Geometry check sheet. Reference: the model listing, model coordinates, mm. Face numbers are marked on the shaded views. Round coordinates to 2 decimals unless told otherwise and drop trailing zeros. Loops run counter-clockwise (first coordinate to the right, second up) from the corner with the lowest first, then second, coordinate; pieces in that order, holes last. Notation, with made-up numbers: (15, 62.5) - (30, 62.5) arc R10 ccw to (30, 75.5) - close; hole circle Ø1 at (88, 1.5). An arc over 180 degrees is marked (long way). Answer in a Markdown table with one row per item. Add a question column.
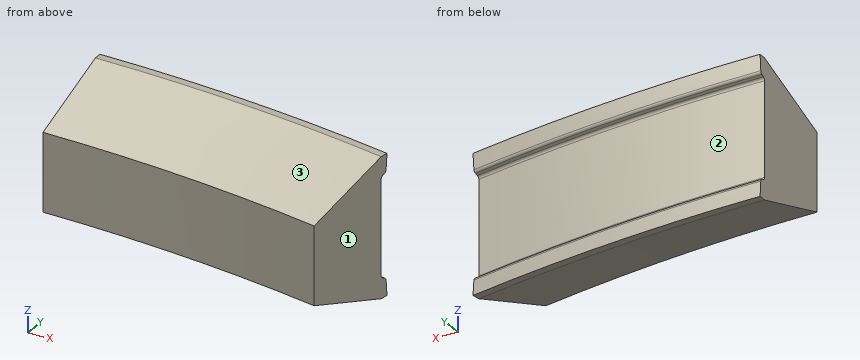
```python
from build123d import *

# Parameters (mm, degrees)
CROQUIS2_R                        = 2.1
CORTAR_EXTRUIR1_DEPTH             = 406.488213274
MATRIZC1_COUNT                    = 36
CORTAR_EXTRUIR5_REACH             = 679.172
CROQUIS4_R                        = 4.2
CORTAR_EXTRUIR5_DIRECTION_2_REACH = 679.172
REVOLUCI_N3_ANGLE                 = 10


with BuildPart() as part:
    # Croquis1 → Revolución2 (revolve)
    with BuildSketch(Plane(origin=(0, 0, 0), x_dir=(0, 0, -1), z_dir=(1, 0, 0)), mode=Mode.PRIVATE) as revoluci_n2_sk:
        with BuildLine():
            Line((-7.932667948, 272.794817661), (-8.128235692, 273.229412649))
            ThreePointArc((-8.128235692, 273.229412649), (-8.296797496, 273.433378016), (-8.545848195, 273.522757553))
            Line((-8.545848195, 273.522757553), (-12.682817286, 273.840985945))
            ThreePointArc((-12.682817286, 273.840985945), (-14.22986011, 274.537339899), (-14.976158002, 276.060917854))
            Line((-14.976158002, 276.060917854), (-16, 285.390918278))
            ThreePointArc((-16, 285.390918278), (-14.380212317, 286.280019748), (-14.896885493, 284.505967215))
            Line((-14.896885493, 284.505967215), (-14.369495262, 279.7))
            ThreePointArc((-14.369495262, 279.7), (-11.00403892, 278.246015718), (-9.3, 275))
            ThreePointArc((-9.3, 275), (-4.661345964, 274.499260763), (0, 274.3))
            ThreePointArc((0, 274.3), (4.661345964, 274.499260763), (9.3, 275))
            ThreePointArc((9.3, 275), (11.00403892, 278.246015718), (14.369495262, 279.7))
            Line((14.369495262, 279.7), (14.896885493, 284.505967215))
            ThreePointArc((14.896885493, 284.505967215), (14.380212317, 286.280019748), (16, 285.390918278))
            Line((16, 285.390918278), (14.976158002, 276.060917854))
            ThreePointArc((14.976158002, 276.060917854), (14.22986011, 274.537339899), (12.682817286, 273.840985945))
            Line((12.682817286, 273.840985945), (8.545848195, 273.522757553))
            ThreePointArc((8.545848195, 273.522757553), (8.296797496, 273.433378016), (8.128235692, 273.229412649))
            Line((8.128235692, 273.229412649), (7.932667948, 272.794817661))
            ThreePointArc((7.932667948, 272.794817661), (7.748192766, 272.580124322), (7.476707195, 272.5))
            Line((7.476707195, 272.5), (-7.476707195, 272.5))
            ThreePointArc((-7.476707195, 272.5), (-7.748192766, 272.580124322), (-7.932667948, 272.794817661))
        make_face()
    revolve(revoluci_n2_sk.sketch.rotate(Axis((0, 0, 417.631684514), (0, 0, -1)), 180), axis=Axis((0, 0, 417.631684514), (0, 0, -1)))

    # Croquis2 → Cortar-Extruir1 (cut, through all)
    with BuildSketch(Plane(origin=(0, 0, 0), x_dir=(1, 0, 0), z_dir=(0, 1, 0))):
        with Locations(Location((0, 0, 0), (0, 0, 270))):
            Circle(CROQUIS2_R)
    cortar_extruir1 = extrude(amount=-CORTAR_EXTRUIR1_DEPTH, mode=Mode.SUBTRACT)

    # MatrizC1: Cortar-Extruir1 ×36 about axis
    matrizc1_axis = Axis((0, 0, 0), (0, 0, 1))
    for i in range(1, MATRIZC1_COUNT):
        add(cortar_extruir1.rotate(matrizc1_axis, i * 360 / MATRIZC1_COUNT), mode=Mode.SUBTRACT)

    # Croquis4 → Cortar-Extruir5 (cut, up to next)
    with BuildSketch(Plane(origin=(-224.693405748, 157.332016491, 0), x_dir=(0, 0, -1), z_dir=(-0.8191520442889971, 0.5735764363510386, 0)), mode=Mode.PRIVATE) as cortar_extruir5_sk1:
        Circle(CROQUIS4_R)
    cortar_extruir5_tool1 = extrude(cortar_extruir5_sk1.sketch, amount=-CORTAR_EXTRUIR5_REACH, mode=Mode.PRIVATE) & part.part
    add(cortar_extruir5_tool1.solids().sort_by_distance((-224.693406, 157.332016, 0))[0], mode=Mode.SUBTRACT)

    # Croquis4 → Cortar-Extruir5 direction 2 (cut, up to next)
    with BuildSketch(Plane(origin=(-224.693405748, 157.332016491, 0), x_dir=(0, 0, -1), z_dir=(-0.8191520442889971, 0.5735764363510386, 0)), mode=Mode.PRIVATE) as cortar_extruir5_direction_2_sk1:
        Circle(CROQUIS4_R)
    cortar_extruir5_direction_2_tool1 = extrude(cortar_extruir5_direction_2_sk1.sketch, amount=CORTAR_EXTRUIR5_DIRECTION_2_REACH, mode=Mode.PRIVATE) & part.part
    add(cortar_extruir5_direction_2_tool1.solids().sort_by_distance((-224.693406, 157.332016, 0))[0], mode=Mode.SUBTRACT)


with BuildPart() as body_2:
    # Croquis5 → Revolución3 (revolve)
    with BuildSketch(Plane(origin=(0, 0, 0), x_dir=(0, 0, -1), z_dir=(1, 0, 0))):
        with BuildLine():
            Line((-11, 273.711538462), (-11, 272.5))
            Line((-11, 272.5), (-7.476707195, 272.5))
            ThreePointArc((-7.476707195, 272.5), (-7.748192766, 272.580124322), (-7.932667948, 272.794817661))
            Line((-7.932667948, 272.794817661), (-8.128235692, 273.229412649))
            ThreePointArc((-8.128235692, 273.229412649), (-8.296797496, 273.433378016), (-8.545848195, 273.522757553))
            Line((-8.545848195, 273.522757553), (-11, 273.711538462))
        make_face()
        Polygon((-7.476707195, 272.5), (-11, 272.5), (-6.179413414, 258.5), (0, 258.5), (0, 272.5), align=None)
        Polygon((7.476707195, 272.5), (0, 272.5), (0, 258.5), (6.179413414, 258.5), (11, 272.5), align=None)
        with BuildLine():
            ThreePointArc((7.932667948, 272.794817661), (7.748192766, 272.580124322), (7.476707195, 272.5))
            Line((7.476707195, 272.5), (11, 272.5))
            Line((11, 272.5), (11, 273.711538462))
            Line((11, 273.711538462), (8.545848195, 273.522757553))
            ThreePointArc((8.545848195, 273.522757553), (8.296797496, 273.433378016), (8.128235692, 273.229412649))
            Line((8.128235692, 273.229412649), (7.932667948, 272.794817661))
        make_face()
    revolve(axis=Axis((0, 0, 417.631684514), (0, 0, -1)), revolution_arc=REVOLUCI_N3_ANGLE)


solid = body_2.part
```
Q1. Scan lines: line 1 (Z direction, x = 21, y = 271.75); line 2 (Z direction, x = 13, y = 266.5); line 3 (Z direction, x = 2, y = 265.75). Record each from-to range of solid material in increasing order. Write a range as from..to.
Q2. Depth check by flat-ended pin: P1, Ø2, axis at x = 37.5, y = 268.5, coming from the -Z side; P2, Ø4, axis at y = 261.5, z = 6.5, coming from the +X side; P3, Ø4, axis at y = 259.5, z = -0.5, coming from the +X side. Enter the tip coordinate at first touch or a pass-through.
Q3. Release check for a two-part mould opening along Z. For the marked faces 1, 2 and 3 record: +Z half, -Z half, draft (parallel to the pull), parting line (faces both ways), or undercut.
Q4. Cross-section at A-A, the plane z = -0.5. Enter the section's corners in (x, y), plus the area to 3 significant figures.
Check sheet entries:
| question | item | result |
|---|---|---|
| 1 | line 1 | -11..-7.71, 7.71..11 |
| 1 | line 2 | -9.04..9.04 |
| 1 | line 3 | -8.68..8.68 |
| 2 | P1 | z = -10.86 |
| 2 | P2 | x = 46.46 |
| 2 | P3 | x = 46.11 |
| 3 | face 1 | draft |
| 3 | face 2 | undercut |
| 3 | face 3 | +Z half |
| 4 | outline | (0, 258.5) arc R258.5 cw to (44.89, 254.57) - (47.32, 268.36) arc R272.5 ccw to (0, 272.5) - close |
| 4 | area | 649 mm² |
